The model under review builds one solid part; all positions refer to its coordinate system, in mm. Round coordinates to 2 decimals unless told otherwise and drop trailing zeros. Order: outer loops, then holes, each group sorted by start corner. A loop starts at its lowest first (then second) coordinate and runs counter-clockwise, first axis right, second up. Notation, with made-up numbers: M 88,46 L 135,46 A25 cw 135,81 Z; hole C -1,65 d3. An arc over 180 degrees is marked long. Answer as a JSON object with one key per item and string values. Group by question number.
1) Consider section D-D, the plane z = 0.4. Write out the cut boundary in (x, y), then the cut area to 3 significant figures.
2) Insertion check: pin 1 Ø3.5 at (y, z) = (2.5, 2) entering from -X; pin 2 Ø1.5 at (x, z) = (-6.5, 1.5) entering from -Y. Each pin has a flat end and moves straight along its axis. Give the tip position at first contact, or say it passes through.
3) Consider section C-C, the plane x = 10. Write out the cut boundary in (y, z), then the cut area to 3 significant figures.
4) Consider section A-A, the plane x = 0. Write out the cut boundary in (y, z).
5) To check wall thickness, follow line 1 (Y direction, x = 0, z = -0.05); line 2 (Y direction, x = 0, z = 1); line 3 (Y direction, x = -8.5, z = 0.7). State the ranges of each line that lie inside material, in increasing order.
Autodesk Inventor part; units mm, degrees
ref_plane "YZ Plane" through (0, 0, 0) normal (1, 0, 0) x (0, 1, 0)
ref_plane "XZ Plane" through (0, 0, 0) normal (0, 1, 0) x (-1, 0, 0)
ref_plane "XY Plane" through (0, 0, 0) normal (0, 0, 1) x (1, 0, 0)
sketch "Sketch1" plane through (0, 0, 0) normal (0, 0, 1) x (1, 0, 0)
  line L0 (14.95, -14.95) -> (-14.95, -14.95)
  line L1 (-14.95, -14.95) -> (-14.95, 14.95)
  line L2 (-14.95, 14.95) -> (14.95, 14.95)
  line L3 (14.95, 14.95) -> (14.95, -14.95)
  line L4 (14.95, -14.95) -> (-14.95, 14.95) construction
  line L5 (-14.95, -14.95) -> (14.95, 14.95) construction
  circle A0 centre (0, 0) radius 0.5
  line L6 (17.45, -17.45) -> (-17.45, -17.45)
  line L7 (-17.45, -17.45) -> (-17.45, 17.45)
  line L8 (-17.45, 17.45) -> (17.45, 17.45)
  line L9 (17.45, 17.45) -> (17.45, -17.45)
  line L10 (17.45, -17.45) -> (-17.45, 17.45) construction
  line L11 (-17.45, -17.45) -> (17.45, 17.45) construction
  dimension "d2" = 29.9
  dimension "d3" = 29.9
  dimension "d4" = 1
  dimension "d5" = 34.9
  dimension "d6" = 34.9
extrude "Extrusion1" add sketch "Sketch1" along normal blind 3 contours L0 L1 L2 L3
extrude "Extrusion2" add sketch "Sketch1" against normal blind 3 contours L0 L1 L2 L3 | L6 L7 L8 L9
properties part number "Large-cuvette-cap-30mm"
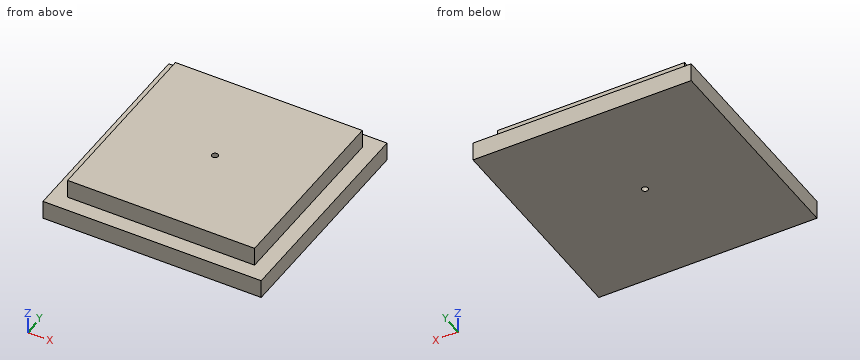
Results list:
{
 "1": {"outline": "M -14.95,-14.95 L 14.95,-14.95 L 14.95,14.95 L -14.95,14.95 Z; hole C 0,0 d1", "area": "893 mm^2"},
 "2": {"pin 1": "x = -14.95", "pin 2": "y = -14.95"},
 "3": {"outline": "M -17.45,-3 L 17.45,-3 L 17.45,0 L 14.95,0 L 14.95,3 L -14.95,3 L -14.95,0 L -17.45,0 Z", "area": "194 mm^2"},
 "4": {"outline": "M -17.45,-3 L -0.5,-3 L -0.5,3 L -14.95,3 L -14.95,0 L -17.45,0 Z; M 0.5,-3 L 17.45,-3 L 17.45,0 L 14.95,0 L 14.95,3 L 0.5,3 Z"},
 "5": {"line 1": "-17.45 to -0.5, 0.5 to 17.45", "line 2": "-14.95 to -0.5, 0.5 to 14.95", "line 3": "-14.95 to 14.95"}
}
